Answer from the drawing. Dimensions are ordinates in mm from the lowest x, y and z of the part. A direction names the side the tool comes from. Give positions to 0.01 mm unless a question says otherwise; leave off trailing zeros. Order: outer loops, then holes, each group sorted by start corner. A loop starts at its lowest first (then second) coordinate and runs counter-clockwise, first axis right, second up. Notation, with made-up numbers: (10.5, 70.5) - (59.5, 70.5) arc R18 cw to (59.5, 79.5) - close; hole circle Ø10 at (54.25, 50). An arc over 180 degrees is marked (long way). Write each question's results on one line, items separated by ' | '.
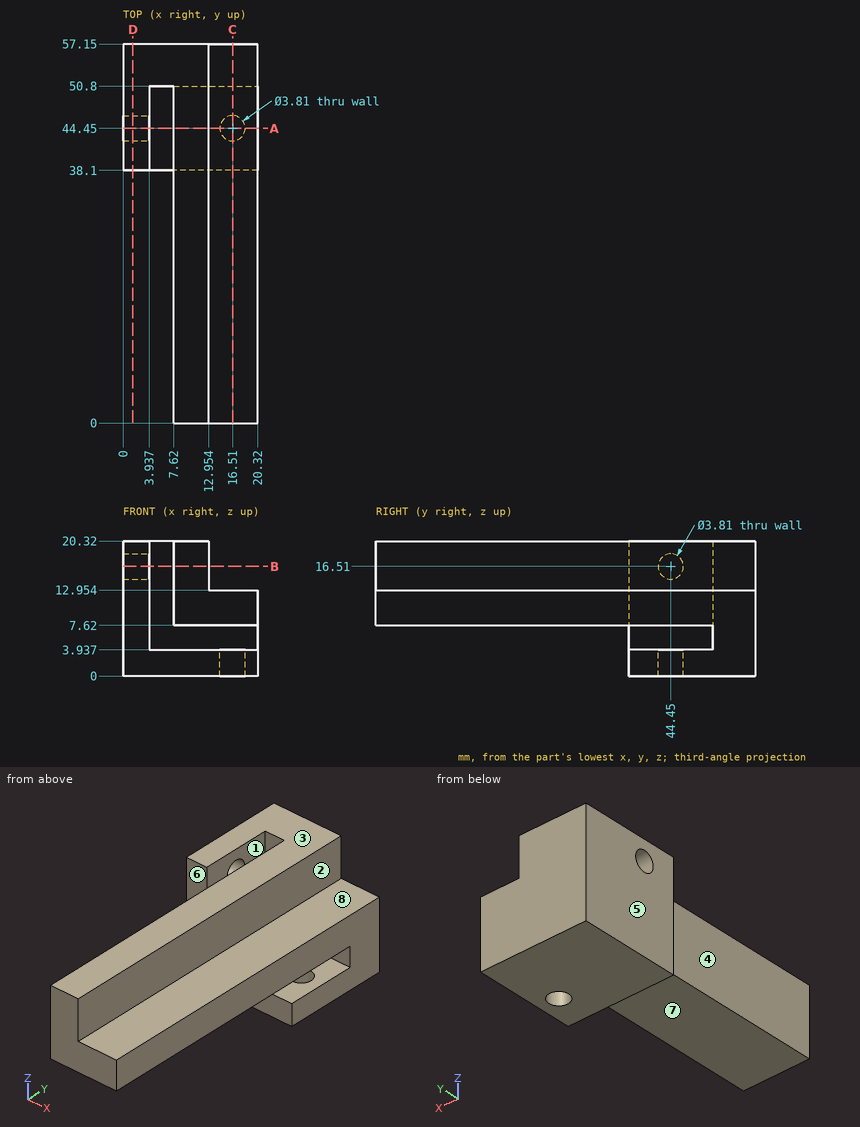
(1) Section D-D (x = 1.5) is taken. Give the vertices of the cut face in (y, z) (3 decimals), plus the area to 3 significant figures.
Conclusion:
outline: (38.1, 0) - (57.15, 0) - (57.15, 20.32) - (38.1, 20.32) - close; hole circle Ø3.81 at (44.45, 16.51) | area: 376 mm^2
(2) Each of these flat-tipped pins is pushed along its axis until it touches: pin 1 (10 mm diameter, centred on x = 15, y = 29.5, fed in from -Z); pin 2 (1.5 mm diameter, centred on x = 6.5, y = 47, fed in from +Z); pin 3 (2.5 mm diameter, centred on y = 44.45, z = 16.51, fed in from -X); pin 4 (6 mm diameter, centred on x = 6, z = 10, fed in from -Y). Where does it stop, or does it pass through?
Conclusion:
pin 1: z = 7.62 | pin 2: z = 3.94 | pin 3: x = 7.62 | pin 4: y = 0
(3) For the marked faces 4, 5, 6, 7 and 8, determine the directions among +Z, -Z, +X, -X, +Y, -Y from which every point of the face is accessible in a straight line to the end or side of a thin tool.
Conclusion:
face 4: +Z, -Y | face 5: +Z, -Z, -X, +Y, -Y | face 6: -Z, -X, -Y | face 7: +X, -Y | face 8: +Z, +X, +Y, -Y
(4) Section C-C (x = 16.51) is taken. Give the vertices of the cut face in (y, z) (3 decimals), plus the area to 3 significant figures.
Conclusion:
outline: (0, 7.62) - (50.8, 7.62) - (50.8, 3.937) - (46.355, 3.937) - (46.355, 0) - (57.15, 0) - (57.15, 12.954) - (0, 12.954) - close; (38.1, 0) - (42.545, 0) - (42.545, 3.937) - (38.1, 3.937) - close | area: 388 mm^2
(5) Section A-A (y = 44.45) is taken. Give the vertices of the cut face in (x, z) (3 decimals).
Conclusion:
outline: (0, 0) - (14.605, 0) - (14.605, 3.937) - (3.937, 3.937) - (3.937, 14.605) - (0, 14.605) - close; (0, 18.415) - (3.937, 18.415) - (3.937, 20.32) - (0, 20.32) - close; (7.62, 7.62) - (20.32, 7.62) - (20.32, 12.954) - (12.954, 12.954) - (12.954, 20.32) - (7.62, 20.32) - close; (18.415, 0) - (20.32, 0) - (20.32, 3.937) - (18.415, 3.937) - close
(6) Consider probe 1 along Y at (x, z) = (1.25, 16.51) (3 decimals); probe 2 along Z at (x, y) = (2.4, 44.45) (3 decimals). Determine where each line is inside the solid, lowest interval first. Write a range as [from, to].
Conclusion:
probe 1: [38.1, 42.545], [46.355, 57.15] | probe 2: [0, 14.605], [18.415, 20.32]
(7) The mould has two halves that part along X. Classify the marked faces 1, 2 and 3: pulls with the +X half, pulls with the -X half, needs draft (parallel to the pull), parting line crosses it, or undercut.
Conclusion:
face 1: undercut | face 2: pulls with the +X half | face 3: needs draft
(8) Section B-B (z = 16.51) is taken. Give the vertices of the cut face in (x, y) (3 decimals), plus the area to 3 significant figures.
Conclusion:
outline: (0, 38.1) - (3.937, 38.1) - (3.937, 42.545) - (0, 42.545) - close; (0, 46.355) - (3.937, 46.355) - (3.937, 50.8) - (7.62, 50.8) - (7.62, 0) - (12.954, 0) - (12.954, 57.15) - (0, 57.15) - close | area: 388 mm^2
